For this review, take the finished solid that the model builds, in its own axes (mm). Face numbers are marked on the shaded views. A direction names the side the tool comes from. Give positions to 0.01 mm unless a question says otherwise; leave off trailing zeros. Loops run counter-clockwise (first coordinate to the right, second up) from the corner with the lowest first, then second, coordinate; pieces in that order, holes last. Notation, with made-up numbers: (3.25, 40) - (61.25, 40) arc R27 cw to (61.25, 67) - close; hole circle Ø11 at (35.5, 28.5). An arc over 180 degrees is marked (long way). Put each result on its own line as item: value.
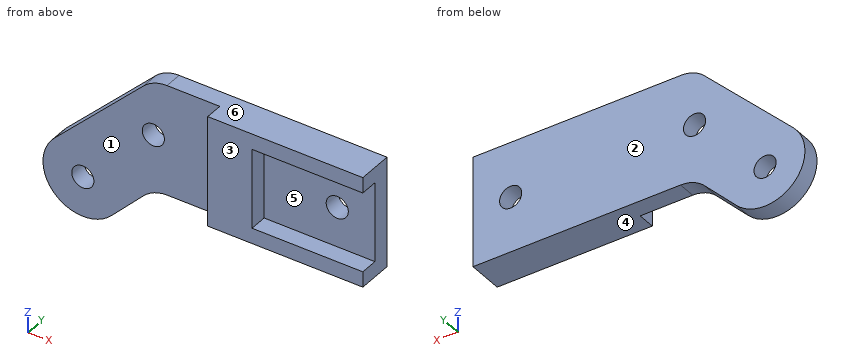
from build123d import *

# Parameters (mm, degrees)
SKETCH1_R           = 5
BOSS_EXTRUDE1_DEPTH = 8
BOSS_EXTRUDE2_DEPTH = 8
FILLET1_R           = 15


with BuildPart() as part:
    # Sketch1 → Boss-Extrude1 (new body)
    with BuildSketch(Plane(origin=(0, 0, 0), x_dir=(1, 0, 0), z_dir=(0, 1, 0))):
        with BuildLine():
            Line((0, -25), (100, -25))
            Line((100, -25), (100, 25))
            Line((100, 25), (0, 25))
            Line((0, 25), (-18.942042706, 44.396101681))
            ThreePointArc((-18.942042706, 44.396101681), (-44.505039362, 44.590272375), (-44.48205564, 19.026548624))
            Line((-44.48205564, 19.026548624), (0, -25))
        make_face()
        with Locations((-31.819805153, 31.819805153)):
            Circle(SKETCH1_R, mode=Mode.SUBTRACT)
        Circle(SKETCH1_R, mode=Mode.SUBTRACT)
        with Locations((83, 0)):
            Circle(SKETCH1_R, mode=Mode.SUBTRACT)
    extrude(amount=BOSS_EXTRUDE1_DEPTH)

    # Sketch2 → Boss-Extrude2 (add)
    with BuildSketch(Plane.XZ):
        Polygon((100, 25), (30, 25), (30, -25), (100, -25), (100, -18), (50, -18), (50, 18), (100, 18), align=None)
    extrude(amount=BOSS_EXTRUDE2_DEPTH)

    # Fillet1
    fillet1_edges = [part.edges().sort_by_distance(p)[0] for p in [
        (0, 4, -25),
        (0, 4, 25),
    ]]
    fillet(fillet1_edges, radius=FILLET1_R)


solid = part.part
1) Insertion check: pin 1 Ø4 at (x, y) = (4, 3) entering from -Z; pin 2 Ø4 at (y, z) = (-3.5, 2.5) entering from +X; pin 3 Ø9 at (y, z) = (-2.5, -11.5) entering from -X; pin 4 Ø6 at (x, y) = (22.5, -2.5) entering from +Z. Each pin has a flat end and moves straight along its axis. Give the tip position at first contact, or say it passes through.
Geometry check:
pin 1: stops at z = -25.63
pin 2: stops at x = 50
pin 3: stops at x = -40.66
pin 4: stops at z = 25
2) Take a section at C-C on z = 0. State the section outline as (x, y) points.
Geometry check:
outline: (-25.26, 0) - (-5, 0) - (-5, 8) - (-25.26, 8) - close; (5, 0) - (30, 0) - (30, -8) - (50, -8) - (50, 0) - (78, 0) - (78, 8) - (5, 8) - close; (88, 0) - (100, 0) - (100, 8) - (88, 8) - close
3) Draft analysis for pull direction Z (two halves, no side actions). For the marked faces 3, 4, 5 and 6, state which applies: pulls with the +Z half, pulls with the -Z half, needs draft (parallel to the pull), parting line crosses it, or undercut.
Geometry check:
face 3: needs draft
face 4: pulls with the -Z half
face 5: undercut
face 6: pulls with the +Z half
4) Take a section at A-A on x = 0. State the section outline as (y, z) points, and give its area (3 significant figures).
Geometry check:
outline: (0, -26.4) - (8, -26.4) - (8, -5) - (0, -5) - close; (0, 5) - (8, 5) - (8, 23.67) - (0, 23.67) - close
area: 321 mm²
5) Take a section at D-D on y = 2.5. State the section outline as (x, z) points.
Geometry check:
outline: (-44.48, -19.03) arc R18 ccw (long way) to (-18.94, -44.4) - (-4.41, -29.52) arc R15 cw to (6.32, -25) - (100, -25) - (100, 25) - (6.17, 25) arc R15 ccw to (-4.38, 20.66) - close; hole circle Ø10 at (-31.82, -31.82); hole circle Ø10 at (0, 0); hole circle Ø10 at (83, 0)
6) Take a section at B-B on y = -5. State the section outline as (x, z) points.
Geometry check:
outline: (30, -25) - (100, -25) - (100, -18) - (50, -18) - (50, 18) - (100, 18) - (100, 25) - (30, 25) - close
7) For the marked faces 1 and 2, list the 3-axis set-ups (+Z, -Z, +X, -X, +Y, -Y) from which the entire face can be reached by the end or side of a thin tool; tool diameter is ignored.
Geometry check:
face 1: +Z, -Z, -X, -Y
face 2: +Z, -Z, +X, -X, +Y
8) Wall thickness on line 1 (Z direction, x = 69, y = -7); line 2 (Z direction, x = 67, y = 2.75); line 3 (Y direction, x = -26.5, z = -11): over which ranges is each line inside the solid? List them lowest first.
Geometry check:
line 1: z = -25 to -18, 18 to 25
line 2: z = -25 to 25
line 3: y = 0 to 8
